For this review, take the finished solid that the model builds, in its own axes (mm). A direction names the side the tool comes from. Give positions to 0.01 mm unless a question says otherwise; leave off trailing zeros. Write each loop counter-clockwise with the first axis right and the second up, starting at its lowest first coordinate (ties: lowest second). Pieces come first, ordered by that corner, then holes. Notation, with made-up numbers: M 45,32 L 74,32 A25 cw 74,58 Z; hole C -17.75,71 d3. An arc over 180 degrees is marked long. Write item = value, one per line.
```python
from build123d import *

# Parameters (mm, degrees)
F0_R     = 40
F0_R_2   = 3.5
F0_R_3   = 1
F0_W     = 40
F0_H     = 40
F1_DEPTH = 5


with BuildPart() as f1:
    # F0 (on Top) → F1 (new body)
    with BuildSketch(Plane.XY):
        Circle(F0_R)
        with Locations((-25.5, 0)):
            Circle(F0_R_2, mode=Mode.SUBTRACT)
        with Locations((-18.5, 23)):
            Circle(F0_R_3, mode=Mode.SUBTRACT)
        Rectangle(F0_W, F0_H, mode=Mode.SUBTRACT)
        with Locations((25.5, 0)):
            Circle(F0_R_2, mode=Mode.SUBTRACT)
        with Locations((18.5, 23)):
            Circle(F0_R_3, mode=Mode.SUBTRACT)
    extrude(amount=F1_DEPTH)


solid = f1.part
```
1. We need section B-B, the plane y = 0. Write out the cut boundary in (x, z), then the cut area to 3 significant figures.
Responses:
outline = M -40,0 L -29,0 L -29,5 L -40,5 Z; M -22,0 L -20,0 L -20,5 L -22,5 Z; M 20,0 L 22,0 L 22,5 L 20,5 Z; M 29,0 L 40,0 L 40,5 L 29,5 Z
area = 130 mm2
2. We need section A-A, the plane z = 2.2. Write out the cut boundary in (x, y).
Responses:
outline = C 0,0 d80; hole C -25.5,0 d7; hole M -20,-20 L 20,-20 L 20,20 L -20,20 Z; hole C -18.5,23 d2; hole C 18.5,23 d2; hole C 25.5,0 d7
3. We need section C-C, the plane x = 0. Write out the cut boundary in (y, z), then the cut area to 3 significant figures.
Responses:
outline = M -40,0 L -20,0 L -20,5 L -40,5 Z; M 20,0 L 40,0 L 40,5 L 20,5 Z
area = 200 mm2
4. The part is to be moulded in two halves that separate along X. For faces 3 (the face through (0, -20, 2)), 4 (the face through (-8.67, -39.05, 2.46)), 5 (the face through (28.84, 1.05, 2.46)), 6 (the face through (-1, -26, 5)), say which applies: +X half, -X half, draft (parallel to the pull), parting line (faces both ways), or undercut.
Responses:
face_3 = undercut
face_4 = parting line
face_5 = undercut
face_6 = draft
5. Insertion check: P1, Ø1, axis at y = -4.5, z = 3, coming from the +X side; P2, Ø2, axis at y = -18, z = 2.5, coming from the -X side; P3, Ø1.6, axis at x = 18.5, y = 23, coming from the -Z side; P4, Ø2.5, axis at x = 3, z = 2.5, coming from the -Y side. Each pin has a flat end and moves straight along its axis. Give the tip position at first contact, or say it passes through.
Responses:
P1 = 39.8
P2 = -36.21
P3 = through
P4 = -39.96
6. For line 1 along Y through (x, z) = (-18.5, 3.5); line 2 along Y through (x, z) = (14.5, 1); line 3 along X through (y, z) = (7, 1.25), list the stretches that pass through material, from the lowest coordinate up. Write a range as from..to.
Responses:
line_1 = -35.46..-20, 20..22, 24..35.46
line_2 = -37.28..-20, 20..37.28
line_3 = -39.38..-20, 20..39.38
7. Machinability: for faces 1 (the face through (-20, 0, 2)), 2 (the face through (-1, -26, 0)), which of the approach directions +Z, -Z, +X, -X, +Y, -Y give a long, thin tool a straight path to every point of the face, cutting with its end or side? Answer none if there is none.
Responses:
face_1 = +Z, -Z
face_2 = -Z, +X, -X, +Y, -Y
8. We need section D-D, the plane y = 23. Write out the cut boundary in (x, z), then the cut area to 3 significant figures.
Responses:
outline = M -32.73,0 L -19.5,0 L -19.5,5 L -32.73,5 Z; M -17.5,0 L 17.5,0 L 17.5,5 L -17.5,5 Z; M 19.5,0 L 32.73,0 L 32.73,5 L 19.5,5 Z
area = 307 mm2
